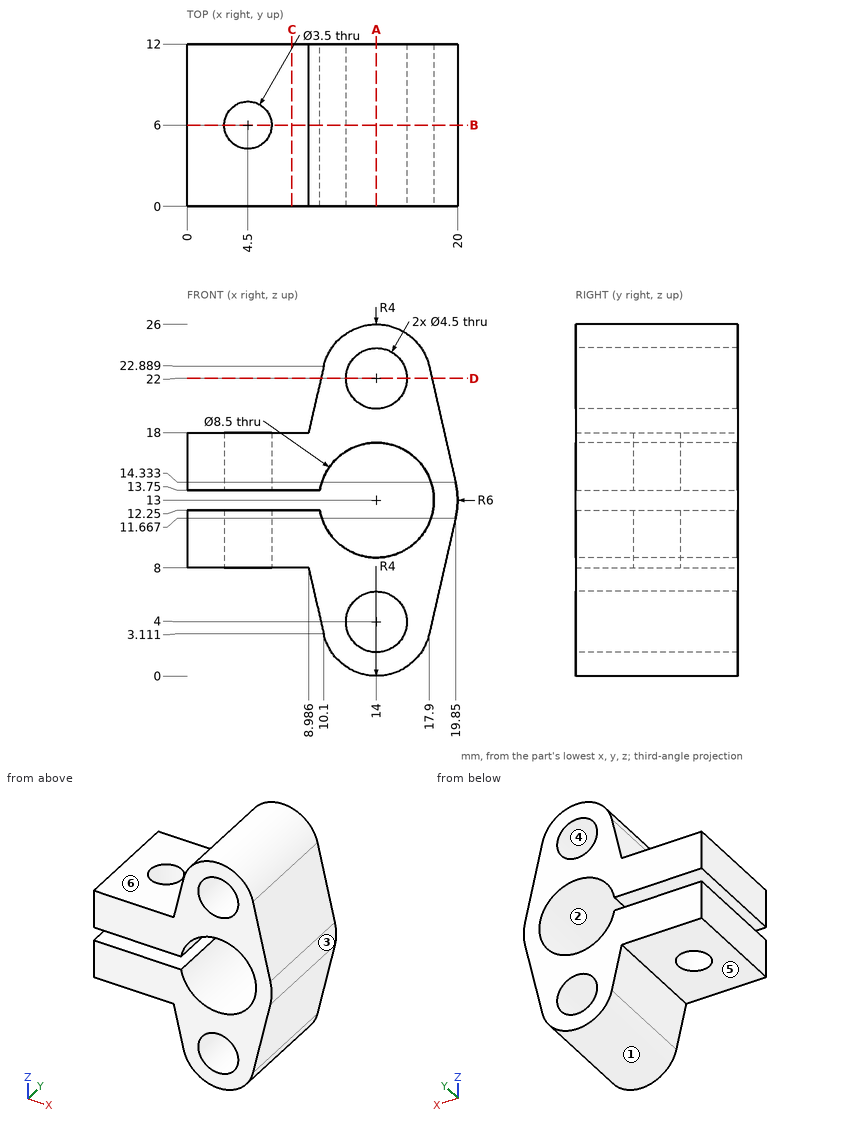
Verification items for this drawing (mm, ordinates from the low corner). A direction names the side the tool comes from. Round coordinates to 2 decimals unless told otherwise and drop trailing zeros. Order: outer loops, then holes, each group sorted by start corner. A loop starts at its lowest first (then second) coordinate and runs counter-clockwise, first axis right, second up. Notation, with made-up numbers: (-36, 66.5) - (8, 66.5) arc R35 cw to (8, 99.5) - close; hole circle Ø2 at (85, -3). An arc over 180 degrees is marked (long way). Use CSV: the item, a comma, the result in double quotes.
(1) Mould release check, pull along Z, two halves, no side actions. Record for the marked faces 1, 2 and 3: released by +Z, released by -Z, zero draft, split by the parting line, or undercut.
Entries:
face 1,"released by -Z"
face 2,"undercut"
face 3,"split by the parting line"
(2) Section check D-D on z = 22. Record the boundary of the cut face in (x, y).
Entries:
outline,"(9.9, 0) - (11.75, 0) - (11.75, 12) - (9.9, 12) - close; (16.25, 0) - (18.1, 0) - (18.1, 12) - (16.25, 12) - close"
(3) Section check C-C on x = 7.75. Record the boundary of the cut face in (y, z), and give its area (3 significant figures).
Entries:
outline,"(0, 8) - (12, 8) - (12, 12.25) - (0, 12.25) - close; (0, 13.75) - (12, 13.75) - (12, 18) - (0, 18) - close"
area,"102 mm^2"
(4) Access from +Z, -Z, +X, -X, +Y, -Y to the whole of each face (thin tool, end or side, straight path). Record for the marked faces 4, 5 and 6.
Entries:
face 4,"+Y, -Y"
face 5,"-Z, -X, +Y, -Y"
face 6,"+Z, -X, +Y, -Y"
(5) Section check B-B on y = 6. Record the boundary of the cut face in (x, z).
Entries:
outline,"(0, 8) - (2.75, 8) - (2.75, 12.25) - (0, 12.25) - close; (0, 13.75) - (2.75, 13.75) - (2.75, 18) - (0, 18) - close; (6.25, 8) - (8.99, 8) - (10.1, 3.11) arc R4 ccw to (17.9, 3.11) - (19.85, 11.67) arc R6 ccw to (19.85, 14.33) - (17.9, 22.89) arc R4 ccw to (10.1, 22.89) - (8.99, 18) - (6.25, 18) - (6.25, 13.75) - (9.82, 13.75) arc R4.25 cw (long way) to (9.82, 12.25) - (6.25, 12.25) - close; hole circle Ø4.5 at (14, 4); hole circle Ø4.5 at (14, 22)"
(6) Section check A-A on x = 14. Record the boundary of the cut face in (y, z), and give its area (3 significant figures).
Entries:
outline,"(0, 0) - (12, 0) - (12, 1.75) - (0, 1.75) - close; (0, 6.25) - (12, 6.25) - (12, 8.75) - (0, 8.75) - close; (0, 17.25) - (12, 17.25) - (12, 19.75) - (0, 19.75) - close; (0, 24.25) - (12, 24.25) - (12, 26) - (0, 26) - close"
area,"102 mm^2"
(7) Gauge pin test, flat ends, axial feed: pin 1 Ø5 at (x, y) = (4, 6.5) entering from -Z; pin 2 Ø8 at (x, z) = (12, 5) entering from -Y; pin 3 Ø3 at (x, y) = (4.5, 6) entering from +Z; pin 4 Ø4.5 at (x, y) = (6, 8.5) entering from +Z. Record the tip position at first contact, or that the pin passes through.
Entries:
pin 1,"z = 8"
pin 2,"y = 0"
pin 3,"through"
pin 4,"z = 18"
(8) Thickness scan on probe 1 along Z at (x, y) = (4.5, 11.25); probe 2 along Z at (x, y) = (12.5, 2) (1 decimal); probe 3 along Y at (x, z) = (4.5, 10.35). Record the ranges inside material, lowest first. Write a range as from..to.
Entries:
probe 1,"8..12.25, 13.75..18"
probe 2,"0.3..2.3, 5.7..9, 17..20.3, 23.7..25.7"
probe 3,"0..4.25, 7.75..12"
